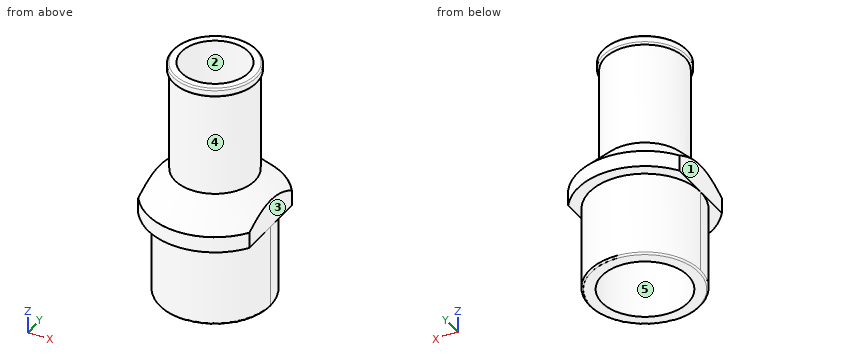
from build123d import *

# Parameters (mm, degrees)
SKETCH061_R          = 6.6
SKETCH061_R_2        = 5.125
PAD009_DEPTH         = 10
SKETCH062_R          = 8
SKETCH062_R_2        = 4
PAD010_DEPTH         = 1.9
SKETCH063_R          = 4.75
SKETCH063_R_2        = 4
PAD011_DEPTH         = 15.5
SKETCH064_R          = 5
SKETCH064_R_2        = 4
PAD012_DEPTH         = 1
CHAMFER_SIZE         = 3.24
FILLET002_R          = 0.2
SKETCH065_W          = 11.246889
SKETCH065_H          = 18.579264
SKETCH065_W_2        = 10.317355
SKETCH065_H_2        = 19.434534
POCKET012_DEPTH      = 100
POCKET012_DEPTH_BACK = 100


with BuildPart() as part:
    # Sketch061 → Pad009 (new body)
    with BuildSketch(Plane.XY):
        Circle(SKETCH061_R)
        Circle(SKETCH061_R_2, mode=Mode.SUBTRACT)
    extrude(amount=PAD009_DEPTH)

    # Sketch062 (on Face4 of Pad009) → Pad010 (join)
    with BuildSketch(Plane.XY.offset(10)):
        Circle(SKETCH062_R)
        Circle(SKETCH062_R_2, mode=Mode.SUBTRACT)
    extrude(amount=PAD010_DEPTH)

    # Sketch063 (on Face7 of Pad010) → Pad011 (join)
    with BuildSketch(Plane.XY.offset(11.9)):
        Circle(SKETCH063_R)
        Circle(SKETCH063_R_2, mode=Mode.SUBTRACT)
    extrude(amount=PAD011_DEPTH)

    # Sketch064 (on Face11 of Pad011) → Pad012 (join)
    with BuildSketch(Plane.XY.offset(27.4)):
        Circle(SKETCH064_R)
        Circle(SKETCH064_R_2, mode=Mode.SUBTRACT)
    extrude(amount=PAD012_DEPTH)

    # Chamfer
    chamfer_edges = [part.edges().sort_by_distance(p)[0] for p in [
        (-4.75, 0, 11.9),
    ]]
    chamfer(chamfer_edges, length=CHAMFER_SIZE)

    # Fillet002
    fillet002_edges = [part.edges().sort_by_distance(p)[0] for p in [
        (-5, 0, 28.4),
        (-5, 0, 27.4),
        (-6.6, 0, 0),
    ]]
    fillet(fillet002_edges, radius=FILLET002_R)

    # Sketch065 → Pocket012 (cut, two sides)
    with BuildSketch(Plane.XZ) as pocket012_sk:
        with Locations((-12.223444, 9.289632)):
            Rectangle(SKETCH065_W, SKETCH065_H)
        with Locations((11.758678, 9.717267)):
            Rectangle(SKETCH065_W_2, SKETCH065_H_2)
    extrude(amount=-POCKET012_DEPTH, mode=Mode.SUBTRACT)
    extrude(pocket012_sk.sketch, amount=POCKET012_DEPTH_BACK, mode=Mode.SUBTRACT)


solid = part.part
Input: part model. Units: mm. Frame: model coordinates. Face numbers are marked on the shaded views. A direction names the side the tool comes from. Coordinates: 2 decimals unless noted, no trailing zeros. Loops run counter-clockwise (first coordinate to the right, second up) from the corner with the lowest first, then second, coordinate; pieces in that order, holes last.
(1) Material intervals for probe 1 along Y at (x, z) = (0, 6.5) (3 decimals); probe 2 along X at (y, z) = (3.5, 15.25); probe 3 along X at (y, z) = (-0.25, 27), sorted ascending.
(2) Pull-direction query (X, two-part tool) for the marked faces 1, 2 and 3; classes: released by +X, released by -X, zero draft, split by the parting line, or undercut.
(3) First-contact query: pin 1 Ø4 at (x, z) = (-5, 22) entering from -Y; pin 2 Ø1.5 at (y, z) = (3, 5.5) entering from +X; pin 3 Ø1.5 at (x, z) = (4, 10.5) entering from -Y. Flat tips, straight axial feed; report the tip coordinate or a pass-through.
(4) Section B-B on z = 21.25. Return the cut outline in (x, y), then the cut area to 3 significant figures.
(5) Set-up query: the marked faces 4 and 5. Return all of +Z, -Z, +X, -X, +Y, -Y with unobstructed straight access to the full face (end or side cutting, diameter ignored); none if empty.
Data:
1. probe 1: y = -6.6 to -5.125, 5.125 to 6.6
1. probe 2: x = -3.21 to -1.94, 1.94 to 3.21
1. probe 3: x = -4.74 to -3.99, 3.99 to 4.74
2. face 1: released by -X
2. face 2: undercut
2. face 3: released by +X
3. pin 1: stops at y = -3.68
3. pin 2: stops at x = 6.2
3. pin 3: stops at y = -7.31
4. outline: circle Ø9.5 at (0, 0); hole circle Ø8 at (0, 0)
4. area: 20.6 mm2
5. face 4: none
5. face 5: -Z
